The model under review builds one solid part; all positions refer to its coordinate system, in mm. Face numbers are marked on the shaded views. A direction names the side the tool comes from. Coordinates: 2 decimals unless noted, no trailing zeros. Write each loop counter-clockwise with the first axis right and the second up, starting at its lowest first coordinate (ties: lowest second). Pieces come first, ordered by that corner, then holes.
1) Add section A-A, the plane x = -3. State the section outline as (y, z) points, then the cut area to 3 significant figures.
2) Machinability: for the marked faces 5 and 6, which of the approach directions +Z, -Z, +X, -X, +Y, -Y give a long, thin tool a straight path to every point of the face, cutting with its end or side? Answer none if there is none.
3) Add section B-B, the plane x = 14. State the section outline as (y, z) points.
4) For line 1 (X direction, y = -3, z = 1); line 2 (Y direction, x = -2.5, z = -1.75); line 3 (Z direction, x = -1.75, y = 0.5), list the stretches that pass through material, from the lowest coordinate up.
5) Mouldability with a two-part tool opening along Z and no side actions: class the marked faces 1, 2, 3 and 4 as released by +Z, released by -Z, zero draft, split by the parting line, or undercut.
6) For P1, Ø2, axis at y = -2.5, z = 0.5, coming from the +X side; P2, Ø2, axis at x = 21.5, y = -3, coming from the -Z side; P3, Ø2, axis at y = 0, z = -1, coming from the -X side, all flat-tipped, find the tip position at first contact; note any pin that passes through.
Autodesk Inventor part; units mm, degrees
ref_plane "Work Plane1" through (29, 0, 0) normal (0, -1, 0) x (1, 0, 0)
ref_plane "YZ Plane" through (0, 0, 0) normal (1, 0, 0) x (0, 1, 0)
ref_plane "XZ Plane" through (0, 0, 0) normal (0, 1, 0) x (-1, 0, 0)
sketch "Sketch1" plane through (0, 0, 0) normal (0, 0, 1) x (1, 0, 0)
  line L0 (-1.1667, 0) -> (25, 0)
  line L1 (25, 0) -> (25, 2.5)
  line L2 (25, 2.5) -> (1.4815, 2.5)
  line L3 (1.4815, 2.5) -> (0.9907, 2.5)
  line L4 (0.9907, 2.5) -> (0, 2.5)
  line L5 (0, 2.5) -> (0, 4.25)
  line L6 (0, 4.25) -> (-5, 4.25)
  line L7 (-5, 4.25) -> (-5, 2.3094)
  line L8 (-5, 2.3094) -> (-2.5, 2.3094)
  line L9 (-2.5, 2.3094) -> (-1.1667, 0)
  line L10 (-11, 0) -> (31, 0)
  line L11 (0, -0.85) -> (0, 5.1)
  line L12 (1.4815, 2.5) -> (0, 2.5) construction
  dimension "d1" = 23.5185
  dimension "d2" = 0.4909
  dimension "d3" = 5
  dimension "d4" = 2.5
  dimension "d5" = 60
  dimension "d6" = 5
  dimension "d7" = 5
  dimension "d8" = 4.6188
  dimension "d9" = 8.5
  dimension "d26" = 25
revolve "Body" add sketch "Sketch1" angle 360 about axis through (-1.1667, 0, 0) along (1, 0, 0)
sketch "Sketch2" plane through (-5, 0, 0) normal (-1, 0, 0) x (0, 0, 1)
  circle A0 centre (0, 0) radius 2.3094
  line L0 (0, -5.95) -> (0, 5.95)
  line L1 (-5.95, 0) -> (5.95, 0)
  line L2 (2.3094, 0) -> (1.1547, -2)
  line L3 (1.1547, -2) -> (-1.1547, -2)
  line L4 (-1.1547, -2) -> (-2.3094, 0)
  line L5 (-2.3094, 0) -> (-1.1547, 2)
  line L6 (-1.1547, 2) -> (1.1547, 2)
  line L7 (1.1547, 2) -> (2.3094, 0)
extrude "Slot" add sketch "Sketch2" against normal up to next contours L7 A0 | A0 L2 | L6 L0 A0 | A0 L0 L3 | L0 L6 A0 | A0 L3 L0 | L4 A0 | A0 L5
fillet "Fillet1" radius 0.5 1 edges at (-5, -4.25, 0)
thread "Thread"
chamfer "Chamfer1" distance 0.4908 distance2 0.4908 1 edges at (25, -2.5, 0) measured on face at (25, 0.6587, -0.3326)
ref_plane "Work Plane1" through (29, 0, 0) normal (0, -1, 0) x (1, 0, 0)
fillet "Fillet2" radius 0.1 1 edges at (0, -2.5, 0)
equation "\"d1\" = GEL"
equation "\"d3\" = KOH"
equation "\"d4\" = INTI"
equation "\"d6\" = GD"
equation "\"d7\" = BDM"
equation "\"d8\" = 1.1547 * SW"
equation "\"d9\" = KOD"
equation "\"d26\" = NLG"
equation "\"d30\" = R"
equation "\"d17\" = RR"
equation "\"d13\" = GEL"
equation "\"d15\" = -0.5 * SPD + 0.5 * GD"
equation "\"d16\" = GUL"
equation "\"GD\" = NND"
equation "\"NLG\" = 25"
equation "\"GEL\" = 23.51848"
equation "\"KOD\" = 8.5"
equation "\"KOH\" = 5"
equation "\"INTI\" = 2.5"
equation "\"GAL\" = 0.61345 * PTC"
equation "\"GUL\" = 0.61345 * PTC"
equation "\"BDM\" = NND"
equation "\"SW\" = 4"
equation "\"RR\" = 0.5"
equation "\"SPD\" = 4.01848"
equation "\"R\" = 0.1"
equation "\"TOA\" = 30deg"
equation "\"THREADDIA\" = 5"
equation "\"PTC\" = 0.8"
equation "\"NND\" = 5"
equation "\"E0\" = 1.155 * SW"
equation "\"GD1\" = THREADDIA - 1.2269 * PTC"
properties part number "ANSI B18.3.1M - M5x0.8 x 25" material "Steel, Mild"
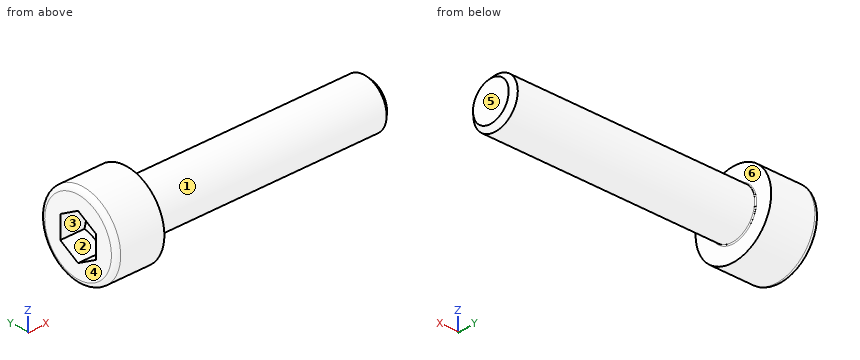
Geometry results:
1. outline: circle Ø8.5 at (0, 0); hole (-2, -1.15) - (0, -2.31) - (2, -1.15) - (2, 1.15) - (0, 2.31) - (-2, 1.15) - close
1. area: 42.9 mm2
2. face 5: +Z, -Z, +X, +Y, -Y
2. face 6: +X
3. outline: circle Ø5 at (0, 0)
4. line 1: x = -5 to 0
4. line 2: y = -3.87 to -0.97, 0.97 to 3.87
4. line 3: z = -4.22 to -0.88, 0.88 to 4.22
5. face 1: split by the parting line
5. face 2: undercut
5. face 3: undercut
5. face 4: zero draft
6. P1: stops at x = 25
6. P2: stops at z = -1.5
6. P3: stops at x = -2.32
